The figure shows three views and two pictorial views of one solid part (mm, origin at its lowest corner). Answer the questions. A direction names the side the tool comes from. Give positions to 0.01 mm unless a question says otherwise; leave off trailing zeros. Order: outer loops, then holes, each group sorted by start corner. A loop starts at its lowest first (then second) coordinate and runs counter-clockwise, first axis right, second up. Notation, with made-up numbers: M 31.5,32 L 80.5,32 A16 cw 80.5,41 Z; hole C 27.5,-32.75 d7. An arc over 180 degrees is marked long. One line per item, written item: value.
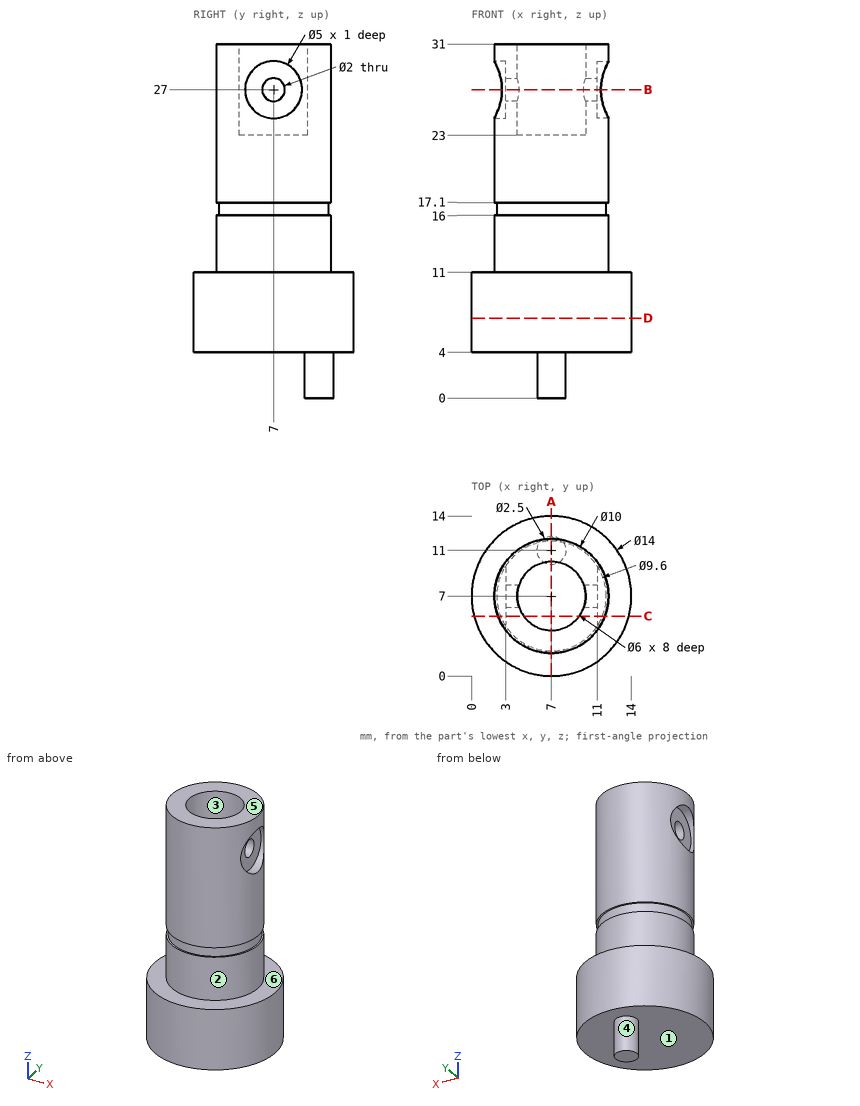
1) Which of the six approach directions +Z, -Z, +X, -X, +Y, -Y give full straight-line access (tool end or side, diameter ignored) to the marked faces 4, 5 and 6?
Reported:
face 4: -Z
face 5: +Z, +X, -X, +Y, -Y
face 6: +Z
2) Consider probe 1 along X at (y, z) = (8, 28); probe 2 along Z at (x, y) = (3.25, 11.5); probe 3 along Z at (x, y) = (10, 10.5). Determine where each line is inside the solid, lowest interval first.
Reported:
probe 1: x = 3 to 4.17, 9.83 to 11
probe 2: z = 4 to 11
probe 3: z = 4 to 31
3) Find section D-D, the plane z = 7. Write down the section's boundary in (x, y).
Reported:
outline: C 7,7 d14
4) Find section C-C, the plane y = 5.25. Write down the section's boundary in (x, z).
Reported:
outline: M 0.22,4 L 13.78,4 L 13.78,11 L 11.68,11 L 11.68,16 L 11.47,16 L 11.47,17.1 L 11.68,17.1 L 11.68,25.21 L 11,25.21 L 11,28.79 L 11.68,28.79 L 11.68,31 L 9.44,31 L 9.44,23 L 4.56,23 L 4.56,31 L 2.32,31 L 2.32,28.79 L 3,28.79 L 3,25.21 L 2.32,25.21 L 2.32,17.1 L 2.53,17.1 L 2.53,16 L 2.32,16 L 2.32,11 L 0.22,11 Z
5) Find section A-A, the plane x = 7. Write down the section's boundary in (y, z).
Reported:
outline: M 0,4 L 9.75,4 L 9.75,0 L 12.25,0 L 12.25,4 L 14,4 L 14,11 L 12,11 L 12,16 L 11.8,16 L 11.8,17.1 L 12,17.1 L 12,31 L 10,31 L 10,23 L 4,23 L 4,31 L 2,31 L 2,17.1 L 2.2,17.1 L 2.2,16 L 2,16 L 2,11 L 0,11 Z
6) Each of these flat-tipped pins is pushed along its axis until it touches: pin 1 Ø2.5 at (y, z) = (6.5, 26.5) entering from +X; pin 2 Ø3 at (x, z) = (4.5, 15.5) entering from +Y; pin 3 Ø6 at (y, z) = (7, 27) entering from -X; pin 4 Ø1.2 at (y, z) = (7, 27) entering from -X (3 decimals). Where does it stop, or does it pass through?
Reported:
pin 1: stops at x = 11
pin 2: stops at y = 11.9
pin 3: stops at x = 2
pin 4: passes through
7) Find section B-B, the plane z = 27. Write down the section's boundary in (x, y), plus the area to 3 significant figures.
Reported:
outline: M 2.67,4.5 A5 ccw 11.33,4.5 L 11,4.5 L 11,6 L 9.83,6 A3 cw 4.17,6 L 3,6 L 3,4.5 Z; M 2.67,9.5 L 3,9.5 L 3,8 L 4.17,8 A3 cw 9.83,8 L 11,8 L 11,9.5 L 11.33,9.5 A5 ccw Z
area: 38.2 mm^2
8) Determine the mould class of the marked faces 1, 2 and 3 for opening direction Y: +Y half, -Y half, draft (parallel to the pull), parting line (faces both ways), or undercut.
Reported:
face 1: draft
face 2: parting line
face 3: undercut
